Geometry: final body of the model. Coordinates: model frame, mm. Face numbers are marked on the shaded views. A direction names the side the tool comes from. Coordinates: 2 decimals unless noted, no trailing zeros. Write each loop counter-clockwise with the first axis right and the second up, starting at its lowest first coordinate (ties: lowest second). Pieces come first, ordered by that corner, then holes. Notation, with made-up numbers: (-34.75, 79.25) -> (-5.75, 79.25) arc R24 ccw to (-5.75, 97.25) -> close; hole circle Ø9 at (61, 51). An arc over 180 degrees is marked (long way). One line per item, written item: value. Start each with the question number.
from build123d import *

# Parameters (mm, degrees)
BOSS_EXTRUDE1_DEPTH = 1.35
CUT_EXTRUDE1_DEPTH  = 16.334791597
CIRPATTERN1_COUNT   = 6
SKETCH5_W           = 2.2
SKETCH5_H           = 4.409341382
BOSS_EXTRUDE2_DEPTH = 1.4


with BuildPart() as part:
    # Sketch1 → Boss-Extrude1 (new body)
    with BuildSketch(Plane.XY):
        Polygon((5.773502692, 10), (-5.773502692, 10), (-11.547005384, 0), (-5.773502692, -10), (5.773502692, -10), (11.547005384, 0), align=None)
    extrude(amount=BOSS_EXTRUDE1_DEPTH)

    # Sketch2 → Cut-Extrude1 (cut, through all)
    with BuildSketch(Plane.XY.offset(1.35)):
        with BuildLine():
            Line((-9.75, 1.75), (-11.547005384, 1.75))
            Line((-11.547005384, 1.75), (-11.547005384, -1.75))
            Line((-11.547005384, -1.75), (-9.75, -1.75))
            ThreePointArc((-9.75, -1.75), (-8, 0), (-9.75, 1.75))
        make_face()
    cut_extrude1 = extrude(amount=-CUT_EXTRUDE1_DEPTH, mode=Mode.SUBTRACT)

    # CirPattern1: Cut-Extrude1 ×6 about axis
    cirpattern1_axis = Axis((0, 0, 0), (0, 0, 1))
    for i in range(1, CIRPATTERN1_COUNT):
        add(cut_extrude1.rotate(cirpattern1_axis, i * 360 / CIRPATTERN1_COUNT), mode=Mode.SUBTRACT)

    # Sketch4 → Revolve1 (revolve)
    with BuildSketch(Plane(origin=(0, 0, 0), x_dir=(1, 0, 0), z_dir=(0, 1, 0)), mode=Mode.PRIVATE) as revolve1_sk:
        with BuildLine():
            Line((-4, -1.35), (-4, -4))
            Line((-4, -4), (-2.75, -4))
            ThreePointArc((-2.75, -4), (-1.858258593, -5.781584453), (0, -6.5))
            Line((0, -6.5), (0, -1.35))
            Line((0, -1.35), (-4, -1.35))
        make_face()
    revolve(revolve1_sk.sketch.rotate(Axis((0, 0, 6.5), (0, 0, -1)), 180), axis=Axis((0, 0, 6.5), (0, 0, -1)))

    # Sketch5 → Boss-Extrude2 (add)
    with BuildSketch(Plane.XY.offset(1.35)):
        with Locations((1.1, 5.545329309)):
            Rectangle(SKETCH5_W, SKETCH5_H)
        with Locations((-1.1, -5.545329309)):
            Rectangle(SKETCH5_W, SKETCH5_H)
    extrude(amount=BOSS_EXTRUDE2_DEPTH)


solid = part.part
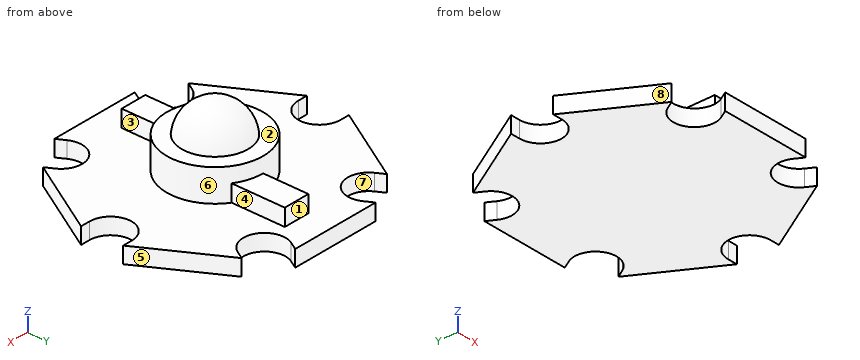
Q1. Draft query along Y for the marked faces 5, 6, 7 and 8. Return one class per face: pulls with the +Y half, pulls with the -Y half, needs draft (parallel to the pull), parting line crosses it, or undercut.
Q2. Line query: L1, parallel to Z at x = -1.5, y = -8.25; L2, parallel to Y at x = -5, z = 1. Output: solid intervals per line, ascending. Write a range as from..to.
Q3. Access query for the marked faces 1, 2, 3 and 4. Directions: +Z, -Z, +X, -X, +Y, -Y. A direction counts if a zero-diameter tool reaches every point of the face in a straight line with its end or side. Return the directions, or none.
Q4. Cut plane A-A on z = 0.75. Output: boundary loops of the cut face in (x, y) (3 decimals).
Q5. Cut plane D-D on z = 2. Output: boundary loops of the cut face in (x, y), and give its area (3 significant figures).
Q6. Cut plane B-B on y = 7.25. Output: boundary loops of the cut face in (x, z).
Q7. First-contact query: P1, Ø1.1, axis at x = 1, y = 6.5, coming from the +Z side; P2, Ø0.7, axis at y = 7, z = 2, coming from the -X side; P3, Ø1.5, axis at y = -0.5, z = 1, coming from the -X side. Flat tips, straight axial feed; report the tip coordinate or a pass-through.
Solution:
1. face 5: pulls with the +Y half
1. face 6: parting line crosses it
1. face 7: undercut
1. face 8: pulls with the -Y half
2. L1: 0..1.35
2. L2: -6.7..6.7
3. face 1: +Z, +X, -X, +Y
3. face 2: +Z
3. face 3: +Z, +X, -Y
3. face 4: +Z, +X, +Y
4. outline: (-10.537, -1.75) -> (-6.784, -8.25) -> (-6.391, -7.569) arc R1.75 cw to (-3.359, -9.319) -> (-3.753, -10) -> (3.753, -10) -> (3.359, -9.319) arc R1.75 cw to (6.391, -7.569) -> (6.784, -8.25) -> (10.537, -1.75) -> (9.75, -1.75) arc R1.75 cw to (9.75, 1.75) -> (10.537, 1.75) -> (6.784, 8.25) -> (6.391, 7.569) arc R1.75 cw to (3.359, 9.319) -> (3.753, 10) -> (-3.753, 10) -> (-3.359, 9.319) arc R1.75 cw to (-6.391, 7.569) -> (-6.784, 8.25) -> (-10.537, 1.75) -> (-9.75, 1.75) arc R1.75 cw to (-9.75, -1.75) -> close
5. outline: (-2.2, -7.75) -> (0, -7.75) -> (0, -4) arc R4 ccw to (2.2, 3.34) -> (2.2, 7.75) -> (0, 7.75) -> (0, 4) arc R4 ccw to (-2.2, -3.34) -> close
5. area: 67.7 mm²
6. outline: (-7.36, 0) -> (-6.15, 0) -> (-6.15, 1.35) -> (-7.36, 1.35) -> close; (-3.6, 0) -> (3.6, 0) -> (3.6, 1.35) -> (2.2, 1.35) -> (2.2, 2.75) -> (0, 2.75) -> (0, 1.35) -> (-3.6, 1.35) -> close; (6.15, 0) -> (7.36, 0) -> (7.36, 1.35) -> (6.15, 1.35) -> close
7. P1: z = 2.75
7. P2: x = 0
7. P3: x = -8.53
